from build123d import *

# Parameters (mm, degrees)
F1_DEPTH = 25
F2_W     = 16.846502
F2_H     = 10.444245
F2_W_2   = 5.885671
F2_H_2   = 9.758566
F3_DEPTH = 1737.001
F5_DEPTH = 80.001
F6_R     = 14
F7_R     = 14
F8_SIZE  = 16
F9_SIZE  = 10


with BuildPart() as f1:
    # F0 (on Front) → F1 (new body)
    with BuildSketch(Plane.XZ):
        Polygon((0, 339.741668), (0, 259.741668), (1737, 259.741668), (1737, 339.741668), (1555, 339.741668), (1555, 320.741668), (585, 320.741668), (585, 339.741668), align=None)
    extrude(amount=F1_DEPTH)

    # F2 (on face) → F3 (cut, through all)
    with BuildSketch(Plane.YZ.offset(1737)):
        with Locations((-25.923251, 257.519545)):
            Rectangle(F2_W, F2_H)
        with Locations((-0.057165, 337.120951)):
            Rectangle(F2_W_2, F2_H_2)
    extrude(amount=-F3_DEPTH, mode=Mode.SUBTRACT)

    # F4 (on face) → F5 (cut, through all)
    with BuildSketch(Plane.XY.offset(339.741668)):
        Polygon((29.025003, -29.025003), (0, 0), (-6.033434, 0), (-6.033434, -29.025003), align=None)
    extrude(amount=-F5_DEPTH, mode=Mode.SUBTRACT)

    # F6
    f6_edges = [f1.edges().sort_by_distance(p)[0] for p in [
        (305, -25, 339.741668),
        (1646, -25, 339.741668),
    ]]
    fillet(f6_edges, radius=F6_R)

    # F7
    f7_edges = [f1.edges().sort_by_distance(p)[0] for p in [
        (1737, -25, 294.241668),
    ]]
    fillet(f7_edges, radius=F7_R)

    # F8
    f8_edges = [f1.edges().sort_by_distance(p)[0] for p in [
        (1070, -25, 320.741668),
    ]]
    chamfer(f8_edges, length=F8_SIZE)

    # F9
    f9_edges = [f1.edges().sort_by_distance(p)[0] for p in [
        (585, -25, 323.241668),
        (1555, -25, 323.241668),
    ]]
    chamfer(f9_edges, length=F9_SIZE)


solid = f1.part
Verification items for the finished model (mm, model axes). Coordinates: 2 decimals unless noted, no trailing zeros. Loops run counter-clockwise (first coordinate to the right, second up) from the corner with the lowest first, then second, coordinate; pieces in that order, holes last. Notation, with made-up numbers: (50.5, -6.75) -> (102.5, -6.75) arc R21 ccw to (102.5, -2.75) -> close; hole circle Ø9 at (2.25, 7). An arc over 180 degrees is marked (long way). Write each question's results on one line, items separated by ' | '.
Item 1: Section check B-B, the plane x = 175.5. Enter the section's corners in (y, z), plus the area to 3 significant figures.
Found:
outline: (-25, 262.74) -> (-17.5, 262.74) -> (-17.5, 259.74) -> (0, 259.74) -> (0, 332.24) -> (-3, 332.24) -> (-3, 339.74) -> (-11, 339.74) arc R14 ccw to (-25, 325.74) -> close | area: 1,910 mm2
Item 2: Gauge pin test, flat ends, axial feed: pin 1 (2.5 mm diameter, centred on x = 364.5, z = 337.5, fed in from +Y); pin 2 (10 mm diameter, centred on x = 1113.5, y = -3, fed in from +Z); pin 3 (2.5 mm diameter, centred on x = 468, z = 260.5, fed in from -Y); pin 4 (3.5 mm diameter, centred on x = 1628.5, y = -1.5, fed in from +Z). Record the tip position at first contact, or that the pin passes through.
Found:
pin 1: stops at y = -3 | pin 2: stops at z = 320.74 | pin 3: stops at y = -17.5 | pin 4: stops at z = 339.74
Item 3: Material ranges on L1, parallel to Z at x = 311.5, y = -13; L2, parallel to Y at x = 640, z = 320.5; L3, parallel to Y at x = 581, z = 330, recorded low to high.
Found:
L1: z = 259.74 to 339.6 | L2: y = -9.24 to 0 | L3: y = -17.77 to 0
Item 4: Section check A-A, the plane x = 1240.5. Enter the section's corners in (y, z).
Found:
outline: (-25, 262.74) -> (-17.5, 262.74) -> (-17.5, 259.74) -> (0, 259.74) -> (0, 320.74) -> (-9, 320.74) -> (-25, 304.74) -> close
